Design review of the part built by this model. Coordinates are the model's own, in mm. Face numbers are marked on the shaded views. A direction names the side the tool comes from. Coordinates: 2 decimals unless noted, no trailing zeros. Write each loop counter-clockwise with the first axis right and the second up, starting at its lowest first coordinate (ties: lowest second). Pieces come first, ordered by that corner, then holes. Notation, with made-up numbers: (-23.75, 65) - (-18.75, 65) arc R20 ccw to (-18.75, 88) - close; hole circle Ø2 at (-26, 19). An arc over 180 degrees is marked (long way). Answer as CSV lines item,"result". Start each with the question number.
Q1. We need section B-B (z = -25). Write out the cut boundary in (x, y), plus the area to 3 significant figures.
Q2. We need section D-D (z = 36.65). Write out the cut boundary in (x, y) (3 decimals).
Q3. Clearance check with flat-ended pins moving along their axes: pin 1 (0.8 mm diameter, centred on x = 1.5, z = -6.5, fed in from +Y); pin 2 (9 mm diameter, centred on x = 13.525, z = 36.65, fed in from +Y); pin 3 (11.5 mm diameter, centred on y = 12, z = -1.5, fed in from +X); pin 4 (1.5 mm diameter, centred on x = 16.5, y = 3.5, fed in from -Z). State where each tip first meets the part, or that it passes through.
Q4. Machinability: for the marked faces 1 and 2, which of the approach directions +Z, -Z, +X, -X, +Y, -Y give a long, thin tool a straight path to every point of the face, cutting with its end or side? Answer none if there is none.
Q5. We need section A-A (y = 12.7). Write out the cut boundary in (x, z), plus the area to 3 significant figures.
Q6. We need section C-C (x = 16.5). Write out the cut boundary in (y, z), plus the area to 3 significant figures.
Q7. For line 1 along X through (y, z) = (1.15, -36.65) (3 decimals); line 2 along Y through (x, z) = (0.55, 25); line 3 along Y through (x, z) = (19.25, -26), list the stretches that pass through material, from the lowest coordinate up. Write a range as [from, to].
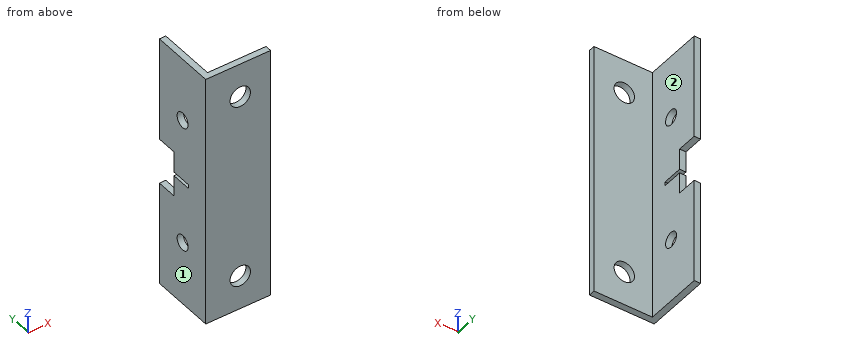
from build123d import *

# Parameters (mm, degrees)
EXTRUDE_THIN1_DEPTH = 50
SKETCH7_R           = 3
CUT_EXTRUDE5_DEPTH  = 62.565574796
CUT_EXTRUDE4_REACH  = 63.566
SKETCH6_R           = 4


with BuildPart() as part:
    # Sketch1 → Extrude-Thin1 (new, symmetric)
    with BuildSketch(Plane.XY):
        Polygon((25.4, 0), (0, 0), (0, 25.4), (2.5, 25.4), (2.5, 2.5), (25.4, 2.5), align=None)
    extrude(amount=EXTRUDE_THIN1_DEPTH, both=True)

    # Sketch7 → Cut-Extrude5 (cut, through all)
    with BuildSketch(Plane.ZY):
        with Locations((-25, 12.7)):
            Circle(SKETCH7_R)
        with Locations((25, 12.7)):
            Circle(SKETCH7_R)
        Polygon((-9, 25.4), (-9, 17.4), (-0.75, 17.4), (-0.75, 9.4), (0.75, 9.4), (0.75, 17.4), (9, 17.4), (9, 25.4), align=None)
    extrude(amount=-CUT_EXTRUDE5_DEPTH, mode=Mode.SUBTRACT)

    # Sketch6 → Cut-Extrude4 (cut, up to next)
    with BuildSketch(Plane.XZ, mode=Mode.PRIVATE) as cut_extrude4_sk1:
        with Locations(Location((13.525, 36.65, 0), (0, 0, 270))):
            Circle(SKETCH6_R)
    cut_extrude4_tool1 = extrude(cut_extrude4_sk1.sketch, amount=-CUT_EXTRUDE4_REACH, mode=Mode.PRIVATE) & part.part
    # Sketch6 → Cut-Extrude4 (cut, up to next)
    with BuildSketch(Plane.XZ, mode=Mode.PRIVATE) as cut_extrude4_sk2:
        with Locations(Location((13.525, -36.65, 0), (0, 0, 270))):
            Circle(SKETCH6_R)
    cut_extrude4_tool2 = extrude(cut_extrude4_sk2.sketch, amount=-CUT_EXTRUDE4_REACH, mode=Mode.PRIVATE) & part.part
    add(cut_extrude4_tool1.solids().sort_by_distance((13.525, 0, 36.65))[0], mode=Mode.SUBTRACT)
    add(cut_extrude4_tool2.solids().sort_by_distance((13.525, 0, -36.65))[0], mode=Mode.SUBTRACT)


solid = part.part
Results list:
1,outline,"(0, 0) - (25.4, 0) - (25.4, 2.5) - (2.5, 2.5) - (2.5, 9.7) - (0, 9.7) - close; (0, 15.7) - (2.5, 15.7) - (2.5, 25.4) - (0, 25.4) - close"
1,area,"106 mm2"
2,outline,"(0, 0) - (9.525, 0) - (9.525, 2.5) - (2.5, 2.5) - (2.5, 25.4) - (0, 25.4) - close; (17.525, 0) - (25.4, 0) - (25.4, 2.5) - (17.525, 2.5) - close"
3,pin 1,"stops at y = 17.4"
3,pin 2,"stops at y = 2.5"
3,pin 3,"stops at x = 2.5"
3,pin 4,"passes through"
4,face 1,"+Z, -Z, -X, +Y, -Y"
4,face 2,"+Z, -Z, +X, +Y"
5,outline,"(0, -50) - (2.5, -50) - (2.5, -28) - (0, -28) - close; (0, -22) - (2.5, -22) - (2.5, -0.75) - (0, -0.75) - close; (0, 0.75) - (2.5, 0.75) - (2.5, 22) - (0, 22) - close; (0, 28) - (2.5, 28) - (2.5, 50) - (0, 50) - close"
5,area,"216 mm2"
6,outline,"(0, -50) - (2.5, -50) - (2.5, -39.32) - (0, -39.32) - close; (0, -33.98) - (2.5, -33.98) - (2.5, 33.98) - (0, 33.98) - close; (0, 39.32) - (2.5, 39.32) - (2.5, 50) - (0, 50) - close"
6,area,"223 mm2"
7,line 1,"x = [0, 9.525], [17.525, 25.4]"
7,line 2,"y = [0, 9.7], [15.7, 25.4]"
7,line 3,"y = [0, 2.5]"
